from build123d import *

# Parameters (mm, degrees)
BOSS_EXTRUDE1_DEPTH = 16
SKETCH2_R           = 0.8
CUT_EXTRUDE1_DEPTH  = 16


with BuildPart() as part:
    # Sketch1 → Boss-Extrude1 (new body)
    with BuildSketch(Plane.XY):
        Polygon((6, 0), (-6, 0), (-6, -5), (-2.5, -5), (-2.5, -4.3), (-2, -3.8), (-2.5, -3.3), (-2.5, -2.3), (2.5, -2.3), (2.5, -3.3), (2, -3.8), (2.5, -4.3), (2.5, -5), (6, -5), align=None)
    extrude(amount=BOSS_EXTRUDE1_DEPTH)

    # Sketch2 → Cut-Extrude1 (cut)
    with BuildSketch(Plane(origin=(0, 0, 0), x_dir=(1, 0, 0), z_dir=(0, 1, 0))):
        with Locations(Location((-4, -8, 0), (0, 0, 270))):
            Circle(SKETCH2_R)
        with Locations(Location((4, -8, 0), (0, 0, 270))):
            Circle(SKETCH2_R)
    extrude(amount=-CUT_EXTRUDE1_DEPTH, mode=Mode.SUBTRACT)


solid = part.part
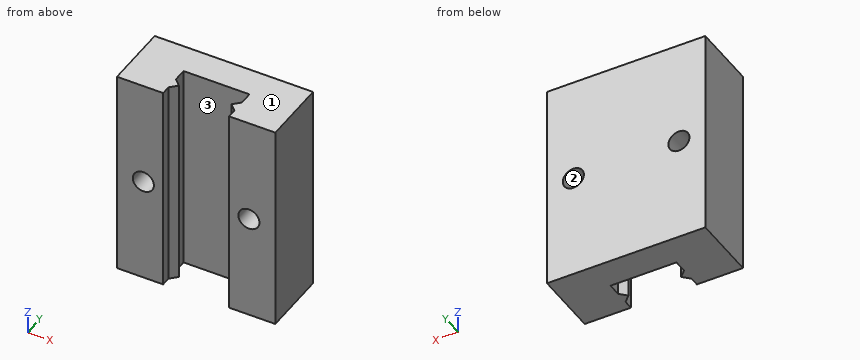
Can you work these out from the model? Positions are in its coordinate system, mm. Face numbers are marked on the shaded views. Round coordinates to 2 decimals unless told otherwise and drop trailing zeros. Order: outer loops, then holes, each group sorted by start corner. A loop starts at its lowest first (then second) coordinate and runs counter-clockwise, first axis right, second up. Notation, with made-up numbers: M 76,79 L 88,79 A19 ccw 88,105 Z; hole C 64.25,61 d10. An arc over 180 degrees is marked long. Use a Markdown table: item, result.
1) Imagine slicing it at B-B (y = -4.55). List the corners of the cut face in (x, z) for me.
Geometry says:
| item | result |
|---|---|
| outline | M -6,0 L -2.5,0 L -2.5,16 L -6,16 Z; M 2.5,0 L 6,0 L 6,16 L 2.5,16 Z; hole C -4,8 d1.6; hole C 4,8 d1.6 |
2) If I drill on line 1 along X through (y, z) = (-1.6, 8); line 2 along X through (y, z) = (-4.5, 1.5); line 3 along X through (y, z) = (-2.55, 8), over which ranges is the centre line in solid material (lowest first)?
Geometry says:
| item | result |
|---|---|
| line 1 | x = -6 to -4.8, -3.2 to 3.2, 4.8 to 6 |
| line 2 | x = -6 to -2.5, 2.5 to 6 |
| line 3 | x = -6 to -4.8, -3.2 to -2.5, 2.5 to 3.2, 4.8 to 6 |
3) Imagine slicing it at D-D (z = 12.5). List the corners of the cut face in (x, y) for me, then the cut area to 3 significant figures.
Geometry says:
| item | result |
|---|---|
| outline | M -6,-5 L -2.5,-5 L -2.5,-4.3 L -2,-3.8 L -2.5,-3.3 L -2.5,-2.3 L 2.5,-2.3 L 2.5,-3.3 L 2,-3.8 L 2.5,-4.3 L 2.5,-5 L 6,-5 L 6,0 L -6,0 Z |
| area | 47.0 mm² |
4) Imagine slicing it at A-A (z = 8). List the corners of the cut face in (x, y) for me.
Geometry says:
| item | result |
|---|---|
| outline | M -6,-5 L -4.8,-5 L -4.8,0 L -6,0 Z; M -3.2,-5 L -2.5,-5 L -2.5,-4.3 L -2,-3.8 L -2.5,-3.3 L -2.5,-2.3 L 2.5,-2.3 L 2.5,-3.3 L 2,-3.8 L 2.5,-4.3 L 2.5,-5 L 3.2,-5 L 3.2,0 L -3.2,0 Z; M 4.8,-5 L 6,-5 L 6,0 L 4.8,0 Z |
5) If we mould it in two halves opening along Z, with no side actions, what happens to the marked faces 1, 2 and 3? For each: +Z half, -Z half, draft (parallel to the pull), parting line (faces both ways), or undercut.
Geometry says:
| item | result |
|---|---|
| face 1 | +Z half |
| face 2 | undercut |
| face 3 | draft |
6) Imagine slicing it at C-C (x = 4). List the corners of the cut face in (y, z) for me.
Geometry says:
| item | result |
|---|---|
| outline | M -5,0 L 0,0 L 0,7.2 L -5,7.2 Z; M -5,8.8 L 0,8.8 L 0,16 L -5,16 Z |
